Geometry: final body of the model. Coordinates: model frame, mm. Face numbers are marked on the shaded views. A direction names the side the tool comes from. Give positions to 0.01 mm unless a question says otherwise; leave off trailing zeros. Write each loop counter-clockwise with the first axis right and the second up, starting at its lowest first coordinate (ties: lowest second). Pieces come first, ordered by that corner, then holes. Notation, with made-up numbers: M 44,80.25 L 63,80.25 A27 ccw 63,98.25 Z; hole C 21.5,24 d6. An arc over 180 degrees is marked long. Answer as a JSON object with one key per item and string values.
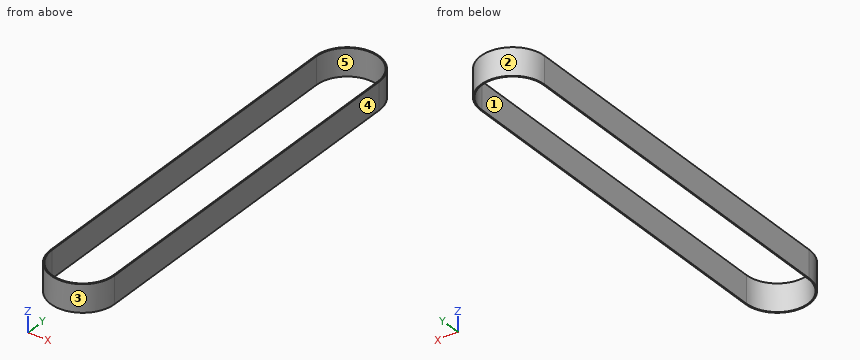
Autodesk Inventor part; units mm, degrees
ref_plane "YZ Plane" through (0, 0, 0) normal (1, 0, 0) x (0, 1, 0)
ref_plane "XZ Plane" through (0, 0, 0) normal (0, 1, 0) x (-1, 0, 0)
ref_plane "XY Plane" through (0, 0, 0) normal (0, 0, 1) x (1, 0, 0)
sketch "Sketch1" plane through (0, 0, 0) normal (0, 0, 1) x (1, 0, 0)
  line L0 (0, 247.65) -> (0, -247.65) construction
  line L1 (-44.45, 247.65) -> (-44.45, -247.65)
  line L2 (44.45, -247.65) -> (44.45, 247.65)
  arc A0 (44.45, 247.65) -> (-44.45, 247.65) centre (0, 247.65) ccw
  arc A1 (-44.45, -247.65) -> (44.45, -247.65) centre (0, -247.65) ccw
  line L3 (-42.8625, -247.65) -> (-42.8625, 247.65)
  arc A2 (42.8625, 247.65) -> (-42.8625, 247.65) centre (0, 247.65) ccw
  line L4 (42.8625, 247.65) -> (42.8625, -247.65)
  arc A3 (-42.8625, -247.65) -> (42.8625, -247.65) centre (0, -247.65) ccw
  point P0 (0, 0)
  dimension "d0" = 495.3
  dimension "d2" = 1.5875
  dimension "d5" = 88.9
extrude "Extrusion1" add sketch "Sketch1" along normal mid plane 38.1
properties part number "1_16 Thick x 1.5 Wide Urethane Flat Belting (10 Long)(217-6001)" material "Rubber"
1) Cut plane C-C on x = 0. Return loops of the section in (y, z), and give its area (3 significant figures).
Geometry check:
{"outline": "M -292.1,-19.05 L -290.51,-19.05 L -290.51,19.05 L -292.1,19.05 Z; M 290.51,-19.05 L 292.1,-19.05 L 292.1,19.05 L 290.51,19.05 Z", "area": "121 mm2"}
2) Cut plane A-A on y = 167. Return loops of the section in (x, z).
Geometry check:
{"outline": "M -44.45,-19.05 L -42.86,-19.05 L -42.86,19.05 L -44.45,19.05 Z; M 42.86,-19.05 L 44.45,-19.05 L 44.45,19.05 L 42.86,19.05 Z"}
3) Line query: line 1 (X direction, y = 227, z = 15.5); line 2 (Y direction, x = -16, z = -12.5); line 3 (Y direction, x = -34, z = 15.5). Output: solid intervals per line, ascending. Write a range as from..to.
Geometry check:
{"line 1": "x = -44.45..-42.86, 42.86..44.45", "line 2": "y = -289.12..-287.41, 287.41..289.12", "line 3": "y = -276.28..-273.75, 273.75..276.28"}
4) Set-up query: the marked faces 1 and 2. Return all of +Z, -Z, +X, -X, +Y, -Y with unobstructed straight access to the full face (end or side cutting, diameter ignored); none if empty.
Geometry check:
{"face 1": "+Z, -Z", "face 2": "+Z, -Z, +Y"}
5) Contact query for flat-ended pins moving along their axis: P1, Ø6, axis at x = 2.5, z = -12.5, coming from the -Y side; P2, Ø1, axis at x = 25, z = 9, coming from the -Y side; P3, Ø5, axis at x = -24.5, z = -1, coming from the -Y side. Output: stop coordinate, or through.
Geometry check:
{"P1": "stops at y = -292.1", "P2": "stops at y = -284.74", "P3": "stops at y = -286.27"}
6) Pull-direction query (X, two-part tool) for the marked faces 3, 4 and 5; classes: pulls with the +X half, pulls with the -X half, needs draft (parallel to the pull), parting line crosses it, or undercut.
Geometry check:
{"face 3": "parting line crosses it", "face 4": "pulls with the +X half", "face 5": "undercut"}
